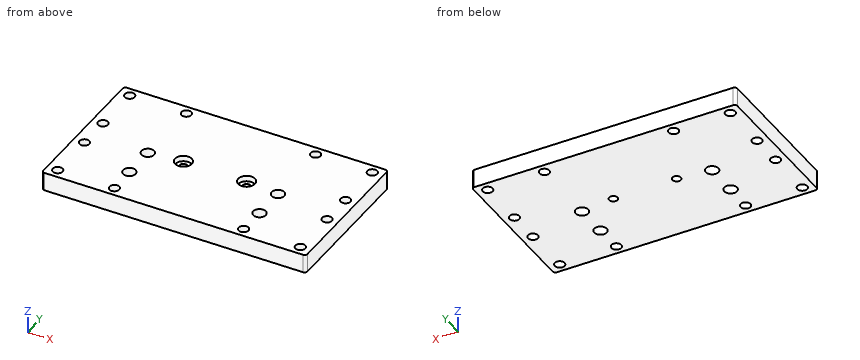
from build123d import *

# Parameters (mm, degrees)
SKETCH1_W                                        = 142
SKETCH1_H                                        = 80
BOSS_EXTRUDE1_DEPTH                              = 5
M5_CLEARANCE_HOLE1_D                             = 5.3
MIRROR2_COPY_1_D                                 = 5.3
CBORE_FOR_M4_PAN_HEAD_MACHINE_SCREW1_D           = 4.5
CBORE_FOR_M4_PAN_HEAD_MACHINE_SCREW1_CBORE_D     = 9
CBORE_FOR_M4_PAN_HEAD_MACHINE_SCREW1_CBORE_DEPTH = 3.1
M8X1_25_TAPPED_HOLE1_D                           = 6.8
FILLET1_R                                        = 1.5


with BuildPart() as part:
    # Sketch1 → Boss-Extrude1 (new body, symmetric)
    with BuildSketch(Plane.XY):
        Rectangle(SKETCH1_W, SKETCH1_H)
    extrude(amount=BOSS_EXTRUDE1_DEPTH, both=True)

    # M5 Clearance Hole1 (through all)
    with Locations(Plane.XY.offset(5)):
        with Locations((-65.25, 35), (-34.75, 35), (-65.25, 9)):
            m5_clearance_hole1 = Hole(M5_CLEARANCE_HOLE1_D / 2)

    # Mirror1: M5 Clearance Hole1 across plane
    add(m5_clearance_hole1.mirror(Plane(origin=(0, 0, 0), x_dir=(0, 0, 1), z_dir=(1, 0, 0))), mode=Mode.SUBTRACT)

    # Mirror2: M5 Clearance Hole1 across plane
    add(m5_clearance_hole1.mirror(Plane.ZX), mode=Mode.SUBTRACT)

    # Mirror2 copy 1 (through all)
    with Locations(Plane(origin=(0, 0, 5), x_dir=(-1, 0, 0), z_dir=(0, 0, 1))):
        with Locations((-65.25, 35), (-34.75, 35), (-65.25, 9)):
            Hole(MIRROR2_COPY_1_D / 2)

    # CBORE for M4 Pan Head Machine Screw1 (through all)
    with Locations(Plane(origin=(-50.308370618, 7.533390419, 5), x_dir=(1, 0, 0), z_dir=(0, 0, 1))):
        with Locations((33.308370618, -7.533390419), (67.308370618, -7.533390419)):
            CounterBoreHole(CBORE_FOR_M4_PAN_HEAD_MACHINE_SCREW1_D / 2, CBORE_FOR_M4_PAN_HEAD_MACHINE_SCREW1_CBORE_D / 2, CBORE_FOR_M4_PAN_HEAD_MACHINE_SCREW1_CBORE_DEPTH)

    # M8x1.25 Tapped Hole1 (through all)
    with Locations(Plane.XY.offset(5)):
        with Locations((-35, -2), (35, -2), (35, -20), (-35, -20)):
            Hole(M8X1_25_TAPPED_HOLE1_D / 2)

    # Fillet1
    fillet1_edges = [part.edges().sort_by_distance(p)[0] for p in [
        (71, -40, 0),
        (-71, -40, 0),
        (-71, 40, 0),
        (71, 40, 0),
    ]]
    fillet(fillet1_edges, radius=FILLET1_R)


solid = part.part
Source: CAD feature listing. Evaluate the final solid. Frame: model axes, mm. Round coordinates to 2 decimals unless told otherwise and drop trailing zeros. Loops run counter-clockwise (first coordinate to the right, second up) from the corner with the lowest first, then second, coordinate; pieces in that order, holes last. Notation, with made-up numbers: (61, -1) -> (94, -1) arc R31 cw to (94, 35) -> close; hole circle Ø2 at (75.25, 54.25). An arc over 180 degrees is marked (long way). Answer as a JSON object with one key per item and string values. Group by question number.
Q1. Section query B-B (x = 65.25). Output: boundary loops of the cut face in (y, z), plus the area to 3 significant figures.
Q2. Contact query for flat-ended pins moving along their axis: P1, Ø5, axis at x = 65.25, y = -35, coming from the +Z side; P2, Ø6, axis at x = -34.75, y = -35, coming from the +Z side; P3, Ø4.5, axis at x = -17, y = -1, coming from the +Z side. Output: stop coordinate, or through.
Q3. Ray query, line 1 (Y direction, x = -65.25, z = 3.25); line 2 (Y direction, x = 34.75, z = 2.25); line 3 (X direction, y = -5, z = -4.25). Return the intervals inside material, ascending. Write a range as from..to.
Q4. Section query C-C (y = -20). Output: boundary loops of the cut face in (x, z).
Q5. Section query D-D (z = 0). State how many separate pieces and enclosed holes the cut face has, plus the area to 3 significant figures.
Q6. Section query A-A (x = -17). Output: boundary loops of the cut face in (y, z), plus the area to 3 significant figures.
Completed:
{
 "1": {"outline": "(-40, -5) -> (-37.65, -5) -> (-37.65, 5) -> (-40, 5) -> close; (-32.35, -5) -> (-11.65, -5) -> (-11.65, 5) -> (-32.35, 5) -> close; (-6.35, -5) -> (6.35, -5) -> (6.35, 5) -> (-6.35, 5) -> close; (11.65, -5) -> (32.35, -5) -> (32.35, 5) -> (11.65, 5) -> close; (37.65, -5) -> (40, -5) -> (40, 5) -> (37.65, 5) -> close", "area": "588 mm²"},
 "2": {"P1": "through", "P2": "z = 5", "P3": "z = 1.9"},
 "3": {"line 1": "-40..-37.65, -32.35..-11.65, -6.35..6.35, 11.65..32.35, 37.65..40", "line 2": "-40..-37.65, -32.35..-23.39, -16.61..-5.39, 1.39..32.35, 37.65..40", "line 3": "-71..-36.6, -33.4..33.4, 36.6..71"},
 "4": {"outline": "(-71, -5) -> (-38.4, -5) -> (-38.4, 5) -> (-71, 5) -> close; (-31.6, -5) -> (31.6, -5) -> (31.6, 5) -> (-31.6, 5) -> close; (38.4, -5) -> (71, -5) -> (71, 5) -> (38.4, 5) -> close"},
 "5": {"separate pieces": "1", "enclosed holes": "18", "area": "10,900 mm²"},
 "6": {"outline": "(-40, -5) -> (-2.25, -5) -> (-2.25, 1.9) -> (-4.5, 1.9) -> (-4.5, 5) -> (-40, 5) -> close; (2.25, -5) -> (40, -5) -> (40, 5) -> (4.5, 5) -> (4.5, 1.9) -> (2.25, 1.9) -> close", "area": "741 mm²"}
}
